from build123d import *

# Parameters (mm, degrees)
SKETCH_1_R      = 2.1
SKETCH_1_R_2    = 3.5
EXTRUDE_2_DEPTH = 3


with BuildPart() as part:
    # 草图1 → 凸台-拉伸2 (new body)
    with BuildSketch(Plane.XY):
        with BuildLine():
            Line((60.108529062, 56.480111122), (64.487335669, 64.669737676))
            ThreePointArc((64.487335669, 64.669737676), (66.140949497, 68.333634007), (67.289887488, 72.185713512))
            Line((67.289887488, 72.185713512), (69.266744251, 80.910498231))
            ThreePointArc((69.266744251, 80.910498231), (68.708488356, 83.415866549), (66.417026795, 84.572466723))
            ThreePointArc((66.417026795, 84.572466723), (64.732022053, 84.734670443), (63.08660729, 85.132365403))
            ThreePointArc((63.08660729, 85.132365403), (54.829995833, 85.201744676), (47.970271321, 80.606026467))
            ThreePointArc((47.970271321, 80.606026467), (43.361470665, 75.124097666), (38.559351744, 69.810695675))
            Line((38.559351744, 69.810695675), (38.222405654, 69.45103511))
            ThreePointArc((38.222405654, 69.45103511), (32.32628292, 64.281621274), (25.53494992, 60.361812759))
            Line((25.53494992, 60.361812759), (-10.053418577, 44.242472458))
            ThreePointArc((-10.053418577, 44.242472458), (-53.239902616, 6.713533173), (-68.783230916, -48.349145956))
            ThreePointArc((-68.783230916, -48.349145956), (-68.739018938, -53.556339201), (-68.762598868, -58.763666747))
            Line((-68.762598868, -58.763666747), (-68.900791413, -71.283477095))
            add(Edge.make_bspline(
                [(-68.900791413, -71.283477095), (-68.904755434, -71.642604913), (-68.869353076, -71.99725933), (-68.78007525, -72.345791606)],
                knots=[0, 0, 0, 0, 1, 1, 1, 1], degree=3))
            Line((-68.78007525, -72.345791606), (-65.332232289, -85.805847824))
            add(Edge.make_bspline(
                [(-65.332232289, -85.805847824), (-65.266290033, -86.063280218), (-65.094030982, -86.28740051), (-64.753434981, -86.484972432), (-64.626638003, -86.528436786), (-64.365301889, -86.564062669), (-64.232742572, -86.556495641), (-64.104070986, -86.52353594)],
                knots=[0, 0, 0, 0, 0.5, 0.5, 0.75, 0.75, 1, 1, 1, 1], degree=3))
            Line((-64.104070986, -86.52353594), (-25.588649762, -76.657668977))
            add(Edge.make_bspline(
                [(-25.588649762, -76.657668977), (-25.460001904, -76.624715354), (-25.338581913, -76.566631903), (-25.128149885, -76.410642035), (-25.037269873, -76.310980591), (-24.901787172, -76.086443416), (-24.85605053, -75.960103889), (-24.81724118, -75.699526051), (-24.823808393, -75.566599434), (-24.856772712, -75.437909819)],
                knots=[0, 0, 0, 0, 0.25, 0.25, 0.5, 0.5, 0.75, 0.75, 1, 1, 1, 1], degree=3))
            Line((-24.856772712, -75.437909819), (-28.008350918, -63.134443476))
            add(Edge.make_bspline(
                [(-28.008350918, -63.134443476), (-28.161648764, -62.535983036), (-28.3702854, -61.960912506), (-28.867938385, -60.844745341), (-29.148955026, -60.300267489), (-29.435424134, -59.758094219)],
                knots=[0, 0, 0, 0, 0.5, 0.5, 1, 1, 1, 1], degree=3))
            ThreePointArc((-29.435424134, -59.758094219), (-29.482770246, -59.668648597), (-29.530246194, -59.579271823))
            add(Edge.make_bspline(
                [(-29.530246194, -59.579271823), (-29.836233344, -59.00420985), (-30.141588994, -58.428815067), (-30.441350493, -57.850472079)],
                knots=[0, 0, 0, 0, 1, 1, 1, 1], degree=3))
            ThreePointArc((-30.441350493, -57.850472079), (-36.012355657, -36.778090759), (-32.088860612, -15.337765675))
            ThreePointArc((-32.088860612, -15.337765675), (-15.685769973, 9.324890383), (8.566391241, 26.329027021))
            Line((8.566391241, 26.329027021), (46.030399371, 43.297916621))
            ThreePointArc((46.030399371, 43.297916621), (54.157658777, 48.726859562), (60.108529062, 56.480111122))
        make_face()
        with Locations((-53.71278904, -79.216483104)):
            Circle(SKETCH_1_R, mode=Mode.SUBTRACT)
        with Locations((-38.213210847, -75.246209079)):
            Circle(SKETCH_1_R, mode=Mode.SUBTRACT)
        with Locations((57.537099808, 74.395494602)):
            Circle(SKETCH_1_R_2, mode=Mode.SUBTRACT)
        Polygon((-56.839024332, -53.987565244), (-54.799481791, -63.777369442), (-45.009677593, -61.737826901), (-47.049220135, -51.948022703), align=None, mode=Mode.SUBTRACT)
        Polygon((-40.670972246, 7.953488017), (-32.543257763, 2.12766127), (-26.717431016, 10.255375753), (-34.845145499, 16.0812025), align=None, mode=Mode.SUBTRACT)
        Polygon((15.066954043, 47.935891978), (19.192847886, 38.826720775), (28.302019088, 42.952614619), (24.176125245, 52.061785821), align=None, mode=Mode.SUBTRACT)
    extrude(amount=EXTRUDE_2_DEPTH)


solid = part.part
Read the model definition and answer for the solid it produces. Units are mm, in the model's axes. A direction names the side the tool comes from. Coordinates: 2 decimals unless noted, no trailing zeros. Order: outer loops, then holes, each group sorted by start corner. A loop starts at its lowest first (then second) coordinate and runs counter-clockwise, first axis right, second up. Notation, with made-up numbers: (-9.75, 85.5) -> (13.25, 85.5) arc R21 cw to (13.25, 108.5) -> close; hole circle Ø7 at (49.5, 30.25). An arc over 180 degrees is marked (long way). Answer as a JSON object with one key per item and string values.
1) The mould has two halves that part along Y. Classify faces 4 (the face through (62.27, 60.52, 1.48)), 5 (the face through (-55.261, -77.797, 1.479)), 6 (the face through (-26, 6, 3)): released by +Y, released by -Y, zero draft, split by the parting line, or undercut.
Model answer:
{"face 4": "released by -Y", "face 5": "undercut", "face 6": "zero draft"}
2) A cutting plane is placed at B-B, the plane y = -30.5. Determine the outline of the cut face in (x, z).
Model answer:
{"outline": "(-67.45, 0) -> (-35.86, 0) -> (-35.86, 3) -> (-67.45, 3) -> close"}
3) Consider line 1 along Y through (x, z) = (-53.5, 2.8); line 2 along Y through (x, z) = (-38, 2.1); line 3 along Y through (x, z) = (20.5, 2.9). Determine where each line is inside the solid, lowest interval first. Write a range as from..to.
Model answer:
{"line 1": "y = -83.81..-81.31, -77.13..-63.51, -53.29..6.3", "line 2": "y = -79.84..-77.34, -73.16..6.04, 11.68..25.34", "line 3": "y = 31.73..39.42, 50.4..58.08"}
4) A cutting plane is placed at A-A, the plane x = 56. Determine the outline of the cut face in (y, z).
Model answer:
{"outline": "(50.61, 0) -> (71.25, 0) -> (71.25, 3) -> (50.61, 3) -> close; (77.54, 0) -> (85.5, 0) -> (85.5, 3) -> (77.54, 3) -> close"}
5) Each of these flat-tipped pins is pushed along its axis until it touches: pin 1 (1.5 mm diameter, centred on x = -22, z = 2, fed in from -Y); pin 2 (3.5 mm diameter, centred on x = -53.71, y = -79.22, fed in from +Z). Where does it stop, or does it pass through?
Model answer:
{"pin 1": "stops at y = 1.02", "pin 2": "passes through"}
6) A cutting plane is placed at C-C, the plane z = 0.9. State how many separate pieces and enclosed holes the cut face has, plus the area to 3 significant figures.
Model answer:
{"separate pieces": "1", "enclosed holes": "6", "area": "5,920 mm²"}
7) A cutting plane is placed at D-D, the plane x = 2.5. Determine the outline of the cut face in (y, z).
Model answer:
{"outline": "(23.26, 0) -> (49.93, 0) -> (49.93, 3) -> (23.26, 3) -> close"}
8) A tool of negligible diameter and unlimited length cuts with its end or side. For faces 1 (the face through (-30.724, 13.128, 1.479)), 2 (the face through (27.036, 34.695, 1.479)), 3 (the face through (-16, 9, 1)), from which of +Z, -Z, +X, -X, +Y, -Y can it reach the whole face along a straight path? Write none if from no direction.
Model answer:
{"face 1": "+Z, -Z", "face 2": "+Z, -Z, +X, -Y", "face 3": "+Z, -Z, +X"}
